Build history of the part. All positions in model axes, mm. A direction names the side the tool comes from. Round coordinates to 2 decimals unless told otherwise and drop trailing zeros. Write each loop counter-clockwise with the first axis right and the second up, starting at its lowest first coordinate (ties: lowest second). Pieces come first, ordered by that corner, then holes. Notation, with made-up numbers: M 79,16 L 106,16 A19 ccw 106,31 Z; hole C -12.5,77 d8. An arc over 180 degrees is marked long. Write item = value, one per line. Start each with the question number.
Q1. Probe L1, parallel to Y at x = 8, z = 7.5; L2, parallel to Y at x = 2, z = 7.5; L3, parallel to Y at x = 18.5, z = 8.25. List the from-to ranges inside material, lowest first.
Q2. Drop flat-ended pins along their axis: P1, Ø3.5, axis at y = 35, z = 7.5, coming from the +X side; P2, Ø6, axis at y = 15, z = 11.5, coming from the -X side; P3, Ø2, axis at y = -5, z = 7.5, coming from the +X side. Give the stop position or say it passes through.
Q3. Band-saw the part on B-B on z = 7.5. Write the cut outline in (x, y), plus the area to 3 significant figures.
Q4. Band-saw the part on D-D on x = 2. Write the cut outline in (y, z).
Q5. Tool access for faces 1 (the cylindrical face through (17.6, 0.6, 14.43)), 2 (the cylindrical face through (17.4, 29.43, 0.6)), 3 (the cylindrical face through (17.6, 0.57, 0.6)), 4 (the cylindrical face through (17.4, 29.4, 14.43)), 5 (the flat face through (18, 30, 7)): list every direction of +Z, -Z, +X, -X, +Y, -Y with a clear straight run to the whole face (end or side of a thin tool).
Q6. Band-saw the part on A-A on y = -5. Write the cut outline in (x, z).
Q7. Band-saw the part on C-C on x = 21. Write the cut outline in (y, z).
Autodesk Inventor part; units mm, degrees
ref_plane "YZ Plane" through (0, 0, 0) normal (1, 0, 0) x (0, 1, 0)
ref_plane "XZ Plane" through (0, 0, 0) normal (0, 1, 0) x (-1, 0, 0)
ref_plane "XY Plane" through (0, 0, 0) normal (0, 0, 1) x (1, 0, 0)
sketch "Sketch1" plane through (0, 0, 0) normal (0, 0, 1) x (1, 0, 0)
  line L0 (0, 0) -> (25, 0)
  line L1 (25, 0) -> (25, 30)
  line L2 (25, 30) -> (0, 30)
  line L3 (0, 30) -> (0, 0)
  circle A0 centre (0, 15) radius 12.2
  point P0 (0, 27.2)
  point P1 (0, 2.8)
  dimension "d0" = 25
  dimension "d1" = 30
  dimension "d2" = 24.4
extrude "Extrusion1" add sketch "Sketch1" along normal blind 15 contours L3 A0 L2 L1 L0
sketch "Sketch2" plane through (0, 30, 0) normal (0, 1, 0) x (1, 0, 0)
  line L0 (0, 0) -> (10, 0)
  line L1 (10, 0) -> (10, -15)
  line L2 (10, -15) -> (0, -15)
  line L3 (0, -15) -> (0, 0)
  dimension "d5" = 10
  dimension "d6" = 15
extrude "Extrusion2" add sketch "Sketch2" along normal blind 10
sketch "Sketch3" plane through (0, 0, 0) normal (0, -1, 0) x (1, 0, 0)
  line L0 (25, 15) -> (10, 15)
  line L1 (0, 0) -> (10, 0)
  line L2 (10, 0) -> (10, 15)
  line L3 (10, 15) -> (0, 15)
  line L4 (0, 15) -> (0, 0)
extrude "Extrusion3" add sketch "Sketch3" along normal blind 10
sketch "Sketch4" plane through (0, 27.2, 0) normal (-1, 0, 0) x (0, 0, 1)
  circle A0 centre (7.5, 7.8) radius 1.4
  line L0 (0, 12.8) -> (0, 0)
  line L1 (0, 12.8) -> (15, 12.8)
  line L2 (0, 0) -> (0, -24.4)
  line L3 (0, -12.2) -> (15, -12.2)
  line L4 (15, -27.2) -> (15, 2.8)
  circle A1 centre (7.5, -32.2) radius 1.4
  point P0 (0, -27.2)
  point P1 (7.5, 12.8)
  dimension "d11" = 2.8
  dimension "d12" = 7.5
  dimension "d13" = 5
extrude "Extrusion4" cut sketch "Sketch4" against normal through all
fillet "Fillet1" radius 2 2 edges at (5, 40, 0) (5, 40, 15)
fillet "Fillet2" radius 2 1 edges at (5, -10, 0)
fillet "Fillet3" radius 2 1 edges at (5, -10, 15)
fillet "Fillet4" radius 2 4 edges at (17.5, 30, 15) (17.5, 30, 0) (17.5, 0, 15) (17.5, 0, 0)
properties part number "motor kapak1"
Conclusion:
q1.L1 = -10 to -6.4, -3.6 to 5.79, 24.21 to 33.6, 36.4 to 40
q1.L2 = -10 to -6.4, -3.6 to 2.97, 27.03 to 33.6, 36.4 to 40
q1.L3 = 0 to 30
q2.P1 = 10
q2.P2 = 11.83
q2.P3 = through
q3.outline = M 0,-10 L 10,-10 L 10,-6.4 L 0,-6.4 Z; M 0,-3.6 L 10,-3.6 L 10,0 L 25,0 L 25,30 L 10,30 L 10,33.6 L 0,33.6 L 0,27.2 A12.2 cw 0,2.8 Z; M 0,36.4 L 10,36.4 L 10,40 L 0,40 Z
q3.area = 660 mm^2
q4.outline = M -10,2 A2 ccw -8,0 L 2.97,0 L 2.97,15 L -8,15 A2 ccw -10,13 Z; M 27.03,0 L 38,0 A2 ccw 40,2 L 40,13 A2 ccw 38,15 L 27.03,15 Z; hole C -5,7.5 d2.8; hole C 35,7.5 d2.8
q5.face_1 = +Z, +X, -Y
q5.face_2 = -Z, +X, +Y
q5.face_3 = -Z, +X, -Y
q5.face_4 = +Z, +X, +Y
q5.face_5 = +Z, -Z, +X, +Y
q6.outline = M 0,0 L 10,0 L 10,6.1 L 0,6.1 Z; M 0,8.9 L 10,8.9 L 10,15 L 0,15 Z
q7.outline = M 0,2 A2 ccw 2,0 L 28,0 A2 ccw 30,2 L 30,13 A2 ccw 28,15 L 2,15 A2 ccw 0,13 Z
